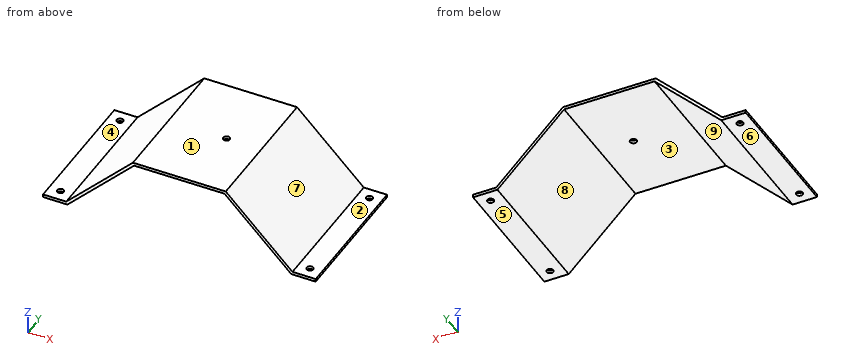
```python
from build123d import *

# Parameters (mm, degrees)
F1_DEPTH = 152.4
F2_R     = 7.1374
F3_DEPTH = 6.351
F5_DEPTH = 152.401


with BuildPart() as f1:
    # F0 (on Front) → F1 (new body, symmetric)
    with BuildSketch(Plane.XZ):
        Polygon((-247.65, -146.05), (-298.45, -146.05), (-298.45, -152.4), (-245.019744, -152.4), (-98.969744, -6.35), (98.969744, -6.35), (245.019744, -152.4), (298.45, -152.4), (298.45, -146.05), (247.65, -146.05), (101.6, 0), (-101.6, 0), align=None)
    extrude(amount=F1_DEPTH, both=True)

    # F2 (on face) → F3 (cut, through all)
    with BuildSketch(Plane.XY.offset(-146.05)):
        with Locations((-273.05, 127)):
            Circle(F2_R)
        with Locations((-273.05, -127)):
            Circle(F2_R)
        with Locations((273.05, 127)):
            Circle(F2_R)
        with Locations((273.05, -127)):
            Circle(F2_R)
    extrude(amount=-F3_DEPTH, mode=Mode.SUBTRACT)

    # F4 (on face) → F5 (cut, through all)
    with BuildSketch(Plane.XY):
        with BuildLine():
            ThreePointArc((32.5374, 0), (25.4, 7.1374), (18.2626, 0))
            Line((18.2626, 0), (32.5374, 0))
        make_face()
        with BuildLine():
            Line((32.5374, 0), (18.2626, 0))
            ThreePointArc((18.2626, 0), (25.4, -7.1374), (32.5374, 0))
        make_face()
    extrude(amount=-F5_DEPTH, mode=Mode.SUBTRACT)


solid = f1.part
```
CAD build for the part. Positions are in the model's coordinates, mm. Face numbers are marked on the shaded views. A direction names the side the tool comes from. Coordinates: 2 decimals unless noted, no trailing zeros. Write each loop counter-clockwise with the first axis right and the second up, starting at its lowest first coordinate (ties: lowest second). Pieces come first, ordered by that corner, then holes. Notation, with made-up numbers: (-30.75, -32) -> (-24.75, -32) arc R22 ccw to (-24.75, -10) -> close; hole circle Ø7 at (31, -31.75). An arc over 180 degrees is marked (long way). Use CSV: the item, a comma, the result in double quotes. Start each with the question number.
Item 1: Band-saw the part on A-A, the plane y = 127. Write the cut outline in (x, z).
Item 2: Band-saw the part on D-D, the plane x = 25.4. Write the cut outline in (y, z).
Item 3: Band-saw the part on C-C, the plane y = 0. Write the cut outline in (x, z), plus the area to 3 significant figures.
Item 4: Two-plate mould, pull along X, no slides. Class the marked faces 6, 7, 8 and 9: +X half, -X half, draft (parallel to the pull), parting line (faces both ways), or undercut.
Item 5: Wall check: probe 1 along Y at (x, z) = (273, -147); probe 2 along Y at (x, z) = (25, -2); probe 3 along Z at (x, y) = (-62, -16). Give the ranges that are in metal, low to high.
Item 6: Band-saw the part on B-B, the plane x = 273.05. Write the cut outline in (y, z), plus the area to 3 significant figures.
Item 7: Tool access for the marked faces 1, 2, 3, 4 and 5: list every direction of +Z, -Z, +X, -X, +Y, -Y with a clear straight run to the whole face (end or side of a thin tool).
Item 8: Drop flat-ended pins along their axis: P1, Ø18.5, axis at x = -273.05, y = 127, coming from the +Z side; P2, Ø23, axis at x = 25.4, y = 0, coming from the -Z side; P3, Ø1.5, axis at x = -137, y = 59.5, coming from the -Z side. Give the stop position or say it passes through.
Response values:
1,outline,"(-298.45, -152.4) -> (-280.19, -152.4) -> (-280.19, -146.05) -> (-298.45, -146.05) -> close; (-265.91, -152.4) -> (-245.02, -152.4) -> (-98.97, -6.35) -> (98.97, -6.35) -> (245.02, -152.4) -> (265.91, -152.4) -> (265.91, -146.05) -> (247.65, -146.05) -> (101.6, 0) -> (-101.6, 0) -> (-247.65, -146.05) -> (-265.91, -146.05) -> close; (280.19, -152.4) -> (298.45, -152.4) -> (298.45, -146.05) -> (280.19, -146.05) -> close"
2,outline,"(-152.4, -6.35) -> (-7.14, -6.35) -> (-7.14, 0) -> (-152.4, 0) -> close; (7.14, -6.35) -> (152.4, -6.35) -> (152.4, 0) -> (7.14, 0) -> close"
3,outline,"(-298.45, -152.4) -> (-245.02, -152.4) -> (-98.97, -6.35) -> (18.26, -6.35) -> (18.26, 0) -> (-101.6, 0) -> (-247.65, -146.05) -> (-298.45, -146.05) -> close; (32.54, -6.35) -> (98.97, -6.35) -> (245.02, -152.4) -> (298.45, -152.4) -> (298.45, -146.05) -> (247.65, -146.05) -> (101.6, 0) -> (32.54, 0) -> close"
3,area,"4,470 mm2"
4,face 6,"draft"
4,face 7,"+X half"
4,face 8,"undercut"
4,face 9,"undercut"
5,probe 1,"y = -152.4 to -134.14, -119.86 to 119.86, 134.14 to 152.4"
5,probe 2,"y = -152.4 to -7.13, 7.13 to 152.4"
5,probe 3,"z = -6.35 to 0"
6,outline,"(-152.4, -152.4) -> (-134.14, -152.4) -> (-134.14, -146.05) -> (-152.4, -146.05) -> close; (-119.86, -152.4) -> (119.86, -152.4) -> (119.86, -146.05) -> (-119.86, -146.05) -> close; (134.14, -152.4) -> (152.4, -152.4) -> (152.4, -146.05) -> (134.14, -146.05) -> close"
6,area,"1,750 mm2"
7,face 1,"+Z, +X, -X, +Y, -Y"
7,face 2,"+Z, +X, +Y, -Y"
7,face 3,"-Z, +Y, -Y"
7,face 4,"+Z, -X, +Y, -Y"
7,face 5,"-Z, +X, -X, +Y, -Y"
8,P1,"stops at z = -146.05"
8,P2,"stops at z = -6.35"
8,P3,"stops at z = -45.13"
